```python
from build123d import *

# Parameters (mm, degrees)
F1_DEPTH = 3
F2_W     = 3
F2_H     = 11
F3_DEPTH = 20


with BuildPart() as f1:
    # F0 (on Top) → F1 (new body)
    with BuildSketch(Plane.XY):
        with BuildLine():
            Line((0, 5.5), (0, 0))
            Line((0, 0), (0, -5.5))
            Line((0, -5.5), (30, -5.5))
            Line((30, -5.5), (30, -2.5))
            Line((30, -2.5), (26, -2.5))
            ThreePointArc((26, -2.5), (22.92305, -2.643382), (21.341688, 0))
            ThreePointArc((21.341688, 0), (22.92305, 2.643382), (26, 2.5))
            Line((26, 2.5), (30, 2.5))
            Line((30, 2.5), (30, 5.5))
            Line((30, 5.5), (0, 5.5))
        make_face()
    extrude(amount=F1_DEPTH)

    # F2 (on face) → F3 (join)
    with BuildSketch(Plane.XY.offset(3)):
        with Locations((1.5, 0)):
            Rectangle(F2_W, F2_H)
    extrude(amount=F3_DEPTH)


solid = f1.part
```
Input: part model. Units: mm. Frame: model coordinates. A direction names the side the tool comes from. Round coordinates to 2 decimals unless told otherwise and drop trailing zeros. Loops run counter-clockwise (first coordinate to the right, second up) from the corner with the lowest first, then second, coordinate; pieces in that order, holes last. Notation, with made-up numbers: (-8, -25.75) -> (20, -25.75) arc R22 cw to (20, 0.25) -> close; hole circle Ø3 at (38.5, 51). An arc over 180 degrees is marked (long way). Use one line per item in the form item = value. Start each with the question number.
Item 1: Contact query for flat-ended pins moving along their axis: pin 1 Ø8 at (x, z) = (10.5, 20) entering from -Y; pin 2 Ø1.5 at (y, z) = (1, 14.5) entering from +X. Output: stop coordinate, or through.
Item 2: Section query D-D on x = 24.25. Return the cut outline in (y, z).
Item 3: Section query B-B on y = 4.25. Return the cut outline in (x, z), then the cut area to 3 significant figures.
Item 4: Mould query, pull axis Y, two halves, no side actions, for faces 1 (the face through (28, 2.5, 1)), 2 (the face through (9, -5.5, 2)), 3 (the face through (0, 0, 11)). Classes: pulls with the +Y half, pulls with the -Y half, needs draft (parallel to the pull), parting line crosses it, or undercut.
Item 5: Section query A-A on x = 28.25. Return the cut outline in (y, z), then the cut area to 3 significant figures.
Item 6: Set-up query: faces 4 (the face through (28, -2.5, 1)), 5 (the face through (30, 4, 1)), 6 (the face through (13, 0, 3)). Return all of +Z, -Z, +X, -X, +Y, -Y with unobstructed straight access to the full face (end or side cutting, diameter ignored); none if empty.
Item 7: Material intervals for L1, parallel to X at y = 0, z = 8.25; L2, parallel to X at y = 0.75, z = 1.25, sorted ascending. Write a range as from..to.
Item 8: Section query C-C on z = 21.25. Return the cut outline in (x, y).
Ans:
q1.pin_1 = through
q1.pin_2 = 3
q2.outline = (-5.5, 0) -> (-3, 0) -> (-3, 3) -> (-5.5, 3) -> close; (3, 0) -> (5.5, 0) -> (5.5, 3) -> (3, 3) -> close
q3.outline = (0, 0) -> (30, 0) -> (30, 3) -> (3, 3) -> (3, 23) -> (0, 23) -> close
q3.area = 150 mm^2
q4.face_1 = undercut
q4.face_2 = pulls with the -Y half
q4.face_3 = needs draft
q5.outline = (-5.5, 0) -> (-2.5, 0) -> (-2.5, 3) -> (-5.5, 3) -> close; (2.5, 0) -> (5.5, 0) -> (5.5, 3) -> (2.5, 3) -> close
q5.area = 18.0 mm^2
q6.face_4 = +Z, -Z, +X
q6.face_5 = +Z, -Z, +X, +Y, -Y
q6.face_6 = +Z, +X, +Y, -Y
q7.L1 = 0..3
q7.L2 = 0..21.44
q8.outline = (0, -5.5) -> (3, -5.5) -> (3, 5.5) -> (0, 5.5) -> close
